from build123d import *

# Parameters (mm, degrees)
BOSS_EXTRUDE1_DEPTH                       = 533.4
CHAMFER1_SIZE                             = 12.7
CSK_FOR_8_FLAT_HEAD_MACHINE_SCREW_2_COUNT = 2
CSK_FOR_8_FLAT_HEAD_MACHINE_SCREW_2_PITCH = 457.2
CSK_FOR_8_FLAT_HEAD_MACHINE_SCREW_3_COUNT = 2
CSK_FOR_8_FLAT_HEAD_MACHINE_SCREW_3_PITCH = 342.9
CSK_FOR_8_FLAT_HEAD_MACHINE_SCREW_4_COUNT = 2
CSK_FOR_8_FLAT_HEAD_MACHINE_SCREW_4_PITCH = 228.6
CSK_FOR_8_FLAT_HEAD_MACHINE_SCREW_5_COUNT = 2
CSK_FOR_8_FLAT_HEAD_MACHINE_SCREW_5_PITCH = 114.3


with BuildPart() as part:
    # Sketch2 → Boss-Extrude1 (new body)
    with BuildSketch(Plane.XY):
        Polygon((0, 0), (0, 50.8), (-3.175, 50.8), (-3.175, 3.175), (-50.8, 3.175), (-50.8, 0), align=None)
    extrude(amount=-BOSS_EXTRUDE1_DEPTH)

    # Chamfer1
    chamfer1_edges = [part.edges().sort_by_distance(p)[0] for p in [
        (-1.5875, 50.8, -533.4),
        (-50.8, 1.5875, -533.4),
        (-50.8, 1.5875, 0),
        (-1.5875, 50.8, 0),
    ]]
    chamfer(chamfer1_edges, length=CHAMFER1_SIZE)

    # Sketch4 → CSK for #8 Flat Head Machine Screw (100)1 (revolve, cut)
    with BuildSketch(Plane(origin=(-26.9875, 3.175, -495.3), x_dir=(0, 0, 1), z_dir=(1, 0, 0))):
        Polygon((0, 0), (0, 3.175), (2.45745, 3.175), (2.45745, 1.475934296), (4.2164, 0), align=None)
    csk_for_8_flat_head_machine_screw_100 = revolve(axis=Axis((-26.9875, 9.525, -495.3), (0, -1, 0)), mode=Mode.SUBTRACT)

    # CSK for _8 Flat Head Machine Screw _ 2: CSK for #8 Flat Head Machine Screw (100)1 ×2
    with Locations(*[(0, 0, i * CSK_FOR_8_FLAT_HEAD_MACHINE_SCREW_2_PITCH) for i in range(1, CSK_FOR_8_FLAT_HEAD_MACHINE_SCREW_2_COUNT)]):
        add(csk_for_8_flat_head_machine_screw_100, mode=Mode.SUBTRACT)

    # CSK for _8 Flat Head Machine Screw _ 3: CSK for #8 Flat Head Machine Screw (100)1 ×2
    with Locations(*[(0, 0, i * CSK_FOR_8_FLAT_HEAD_MACHINE_SCREW_3_PITCH) for i in range(1, CSK_FOR_8_FLAT_HEAD_MACHINE_SCREW_3_COUNT)]):
        add(csk_for_8_flat_head_machine_screw_100, mode=Mode.SUBTRACT)

    # CSK for _8 Flat Head Machine Screw _ 4: CSK for #8 Flat Head Machine Screw (100)1 ×2
    with Locations(*[(0, 0, i * CSK_FOR_8_FLAT_HEAD_MACHINE_SCREW_4_PITCH) for i in range(1, CSK_FOR_8_FLAT_HEAD_MACHINE_SCREW_4_COUNT)]):
        add(csk_for_8_flat_head_machine_screw_100, mode=Mode.SUBTRACT)

    # CSK for _8 Flat Head Machine Screw _ 5: CSK for #8 Flat Head Machine Screw (100)1 ×2
    with Locations(*[(0, 0, i * CSK_FOR_8_FLAT_HEAD_MACHINE_SCREW_5_PITCH) for i in range(1, CSK_FOR_8_FLAT_HEAD_MACHINE_SCREW_5_COUNT)]):
        add(csk_for_8_flat_head_machine_screw_100, mode=Mode.SUBTRACT)


solid = part.part
Build history of the part. All positions in model axes, mm. A direction names the side the tool comes from. Give positions to 0.01 mm unless a question says otherwise; leave off trailing zeros. Order: outer loops, then holes, each group sorted by start corner. A loop starts at its lowest first (then second) coordinate and runs counter-clockwise, first axis right, second up. Notation, with made-up numbers: M -37.5,63.5 L -4.5,63.5 A25 cw -4.5,102.5 Z; hole C 21,85.5 d6. An arc over 180 degrees is marked long. Use one line per item in the form item = value.
Q1. Pin check, flat tips, straight feed: P1, Ø2, axis at x = -19.5, z = -390, coming from the +Y side (3 decimals); P2, Ø10, axis at y = 13, z = -209, coming from the -X side (3 decimals); P3, Ø4.5, axis at x = -26.99, z = -266.7, coming from the +Y side. Stop position of each tip, or through.
Conclusion:
P1 = 3.175
P2 = -3.175
P3 = through
Q2. Slice it at B-B, the plane y = 19.5. Write the cut outline in (x, z) (3 decimals), and give its area (3 significant figures).
Conclusion:
outline = M -3.175,-533.4 L 0,-533.4 L 0,0 L -3.175,0 Z
area = 1,690 mm2
Q3. Pull direction Z, two halves, no side cores. Call faces 3 (the flat face through (-1.6, 44.4, -527.1)), 4 (the flat face through (-3.175, 27, -263)), 5 (the flat face through (-11, 2, 0)): released by +Z, released by -Z, zero draft, split by the parting line, or undercut.
Conclusion:
face_3 = released by -Z
face_4 = zero draft
face_5 = released by +Z
Q4. Wall check: probe 1 along X at (y, z) = (0.85, -381); probe 2 along Y at (x, z) = (-29.5, -330) (3 decimals); probe 3 along X at (y, z) = (32.5, -446.5) (3 decimals). Give the ranges that are in metal, low to high.
Conclusion:
probe_1 = -50.8 to -29.44, -24.53 to 0
probe_2 = 0 to 3.175
probe_3 = -3.175 to 0
Q5. Slice it at A-A, the plane z = -317. Write the cut outline in (x, y) (3 decimals).
Conclusion:
outline = M -50.8,0 L 0,0 L 0,50.8 L -3.175,50.8 L -3.175,3.175 L -50.8,3.175 Z
Q6. Which spindle directions (+Z, -Z, +X, -X, +Y, -Y) get a long thin tool onto all of the face, cutting with end or side? Do faces 1 (the flat face through (-32, 3.175, -263)), 2 (the flat face through (-44.4, 1.6, -6.3)). Say none if no direction does.
Conclusion:
face_1 = +Z, -Z, -X, +Y
face_2 = +Z, -X, +Y, -Y
